Input: part model. Units: mm. Frame: model coordinates. A direction names the side the tool comes from. Give positions to 0.01 mm unless a question says otherwise; leave off trailing zeros. Order: outer loops, then holes, each group sorted by start corner. A loop starts at its lowest first (then second) coordinate and runs counter-clockwise, first axis right, second up.
```python
from build123d import *

# Parameters (mm, degrees)
SKETCH2_R                  = 4
CUT_EXTRUDE1_DEPTH         = 36.832945734
CHAMFER1_SIZE              = 1
M4X0_7_TAPPED_HOLE1_REACH  = 41.314
M4X0_7_TAPPED_HOLE1_BORE_R = 1.65
CIRPATTERN3_COUNT          = 2
CIRPATTERN3_ANGLE          = 120


with BuildPart() as part:
    # Sketch1 → Revolve1 (revolve)
    with BuildSketch(Plane.XY):
        Polygon((0, 10), (20, 10), (20, 0), (10, 0), (10, -12), (0, -12), align=None)
    revolve(axis=Axis((0, -12, 0), (0, 1, 0)))

    # Sketch2 → Cut-Extrude1 (cut, through all)
    with BuildSketch(Plane(origin=(0, 10, 0), x_dir=(1, 0, 0), z_dir=(0, 1, 0))):
        with Locations(Location((0, 0, 0), (0, 0, 180))):
            Circle(SKETCH2_R)
    extrude(amount=-CUT_EXTRUDE1_DEPTH, mode=Mode.SUBTRACT)

    # Chamfer1
    chamfer1_edges = [part.edges().sort_by_distance(p)[0] for p in [
        (-10, -12, 0),
        (-20, 0, 0),
        (-20, 10, 0),
    ]]
    chamfer(chamfer1_edges, length=CHAMFER1_SIZE)

    # M4x0.7 Tapped Hole1 bore (on position points) → M4x0.7 Tapped Hole1 (cut, up to next)
    with BuildSketch(Plane(origin=(-0.085304599, -5.563796066, -9.99963615), x_dir=(-0.999963614965, 0, 0.008530459937), z_dir=(-0.008530459937, 0, -0.999963614965)), mode=Mode.PRIVATE) as m4x0_7_tapped_hole1_sk1:
        Circle(M4X0_7_TAPPED_HOLE1_BORE_R)
    m4x0_7_tapped_hole1_tool1 = extrude(m4x0_7_tapped_hole1_sk1.sketch, amount=-M4X0_7_TAPPED_HOLE1_REACH, mode=Mode.PRIVATE) & part.part
    m4x0_7_tapped_hole1 = m4x0_7_tapped_hole1_tool1.solids().sort_by_distance((-0.085305, -5.563796, -9.999636))[0]
    add(m4x0_7_tapped_hole1, mode=Mode.SUBTRACT)

    # CirPattern3: M4x0.7 Tapped Hole1 ×2 about axis
    cirpattern3_axis = Axis((0, -12, 0), (0, -1, 0))
    for i in range(1, CIRPATTERN3_COUNT):
        add(m4x0_7_tapped_hole1.rotate(cirpattern3_axis, i * CIRPATTERN3_ANGLE / (CIRPATTERN3_COUNT - 1)), mode=Mode.SUBTRACT)


solid = part.part
```
1) Reachability of faces 5 (the face through (-4.336, 4.944, 19.524)), 6 (the face through (-8, -6, 6)) from +Z, -Z, +X, -X, +Y, -Y: full face, straight path, thin tool, end or side. Return the list, or none.
2) Cut plane B-B (x = 0). Count the separate pieces of the cut face and the enclosed holes in it, then the cut area to 3 significant figures.
3) Line query: probe 1 along Z at (x, y) = (0, -2.5); probe 2 along Y at (x, z) = (12.5, 2.5); probe 3 along Z at (x, y) = (0, -6). Output: solid intervals per line, ascending.
4) Pull-direction query (Y, two-part tool) for faces 1 (the face through (8, 0, 8)), 2 (the face through (-3.815, -0.846, 1.201)), 3 (the face through (0.3, 10, -4.5)), 4 (the face through (-0.82, -7.028, -6.86)); classes: pulls with the +Y half, pulls with the -Y half, needs draft (parallel to the pull), parting line crosses it, or undercut.
5) First-contact query: P1, Ø4, axis at x = -14, y = -1.5, coming from the -Z side; P2, Ø2, axis at y = -6.5, z = 12.5, coming from the -X side; P3, Ø4, axis at y = 7, z = -0.5, coming from the -X side; P4, Ø1.5, axis at x = 5, y = -3, coming from the -Z side. Flat tips, straight axial feed; report the tip coordinate or a pass-through.
6) Cut plane A-A (y = -3.25). Return the cut outline in (x, z), then the cut area to 3 significant figures.
Geometry says:
1. face 5: +Y, -Y
1. face 6: -Y
2. separate pieces: 3
2. enclosed holes: 0
2. area: 441 mm2
3. probe 1: z = -10 to -4, 4 to 10
3. probe 2: y = 0 to 10
3. probe 3: z = 4 to 10
4. face 1: pulls with the -Y half
4. face 2: needs draft
4. face 3: pulls with the +Y half
4. face 4: undercut
5. P1: stops at z = -14.18
5. P2: passes through
5. P3: stops at x = -20
5. P4: stops at z = -9.05
6. outline: circle Ø20 at (0, 0); hole circle Ø8 at (0, 0)
6. area: 264 mm2
